Check sheet for the modelled part. Datum: model origin and axes. Units: mm. Face numbers are marked on the shaded views. A direction names the side the tool comes from. Coordinates: 2 decimals unless noted, no trailing zeros. Loops run counter-clockwise (first coordinate to the right, second up) from the corner with the lowest first, then second, coordinate; pieces in that order, holes last.
```python
from build123d import *

# Parameters (mm, degrees)
SKETCH1_W                = 72
SKETCH1_H                = 70
BOSS_EXTRUDE1_DEPTH      = 2
BOSS_EXTRUDE2_DEPTH      = 34
BOSS_EXTRUDE2_DEPTH_BACK = 34
CUT_EXTRUDE1_START       = -34
SKETCH3_W                = 39.5
SKETCH3_H                = 2
CUT_EXTRUDE1_DEPTH       = 68
BOSS_EXTRUDE3_DEPTH      = 2
FILLET2_R                = 1
FILLET2_OF_MIRROR1_R     = 1


with BuildPart() as part:
    # Sketch1 → Boss-Extrude1 (new body)
    with BuildSketch(Plane(origin=(0, 0, 0), x_dir=(1, 0, 0), z_dir=(0, 1, 0))):
        Rectangle(SKETCH1_W, SKETCH1_H)
    extrude(amount=BOSS_EXTRUDE1_DEPTH)

    # Sketch2 → Boss-Extrude2 (add, two sides: drawn at the far end of the back side and taken through both)
    with BuildSketch(Plane(origin=(0, 0, 0), x_dir=(0, 0, -1), z_dir=(1, 0, 0)).offset(-BOSS_EXTRUDE2_DEPTH_BACK)):
        with BuildLine():
            Line((-25.991933385, 2), (-19.75, 2))
            Line((-19.75, 2), (-19.75, 6.5))
            ThreePointArc((-19.75, 6.5), (-13.763212024, 15.155284356), (-3.552389776, 12.606816862))
            Line((-3.552389776, 12.606816862), (3.552389776, 12.606816862))
            ThreePointArc((3.552389776, 12.606816862), (13.763212024, 15.155284356), (19.75, 6.5))
            Line((19.75, 6.5), (19.75, 2))
            Line((19.75, 2), (25.991933385, 2))
            ThreePointArc((25.991933385, 2), (22.513891667, 3.407893959), (20.994535519, 6.838709677))
            ThreePointArc((20.994535519, 6.838709677), (15.537625909, 15.712617717), (5.12195122, 15.51812571))
            ThreePointArc((5.12195122, 15.51812571), (0, 14.106816862), (-5.12195122, 15.51812571))
            ThreePointArc((-5.12195122, 15.51812571), (-15.537625909, 15.712617717), (-20.994535519, 6.838709677))
            ThreePointArc((-20.994535519, 6.838709677), (-22.513891667, 3.407893959), (-25.991933385, 2))
        make_face()
    extrude(amount=BOSS_EXTRUDE2_DEPTH + BOSS_EXTRUDE2_DEPTH_BACK)

    # Sketch3 → Cut-Extrude1 (cut)
    with BuildSketch(Plane(origin=(0, 0, 0), x_dir=(0, 0, -1), z_dir=(1, 0, 0)).offset(CUT_EXTRUDE1_START)):
        with Locations((0, 1)):
            Rectangle(SKETCH3_W, SKETCH3_H)
    extrude(amount=CUT_EXTRUDE1_DEPTH, mode=Mode.SUBTRACT)

    # Sketch4 → Boss-Extrude3 (add)
    with BuildSketch(Plane(origin=(34, 0, 0), x_dir=(0, 0, -1), z_dir=(1, 0, 0))):
        with BuildLine():
            Line((-25.991933385, 2), (25.991933385, 2))
            ThreePointArc((25.991933385, 2), (22.513891667, 3.407893959), (20.994535519, 6.838709677))
            ThreePointArc((20.994535519, 6.838709677), (15.537625909, 15.712617717), (5.12195122, 15.51812571))
            ThreePointArc((5.12195122, 15.51812571), (0, 14.106816862), (-5.12195122, 15.51812571))
            ThreePointArc((-5.12195122, 15.51812571), (-15.537625909, 15.712617717), (-20.994535519, 6.838709677))
            ThreePointArc((-20.994535519, 6.838709677), (-22.513891667, 3.407893959), (-25.991933385, 2))
        make_face()
    boss_extrude3 = extrude(amount=BOSS_EXTRUDE3_DEPTH)

    # Fillet2
    fillet2_edges = [part.edges().sort_by_distance(p)[0] for p in [
        (36, 2, 30.495966692),
        (36, 2, -30.495966692),
        (36, 3.407893959, -22.513891667),
        (36, 15.712617717, -15.537625909),
        (36, 14.106816862, 0),
        (36, 15.712617717, 15.537625909),
        (36, 3.407893959, 22.513891667),
    ]]
    fillet(fillet2_edges, radius=FILLET2_R)

    # Mirror1: Boss-Extrude3 across plane
    add(boss_extrude3.mirror(Plane(origin=(0, 0, 0), x_dir=(0, 0, 1), z_dir=(1, 0, 0))))

    # Fillet2 of Mirror1
    fillet2_of_mirror1_edges = [part.edges().sort_by_distance(p)[0] for p in [
        (-36, 2, 30.495966692),
        (-36, 2, -30.495966692),
        (-36, 3.407893959, -22.513891667),
        (-36, 15.712617717, -15.537625909),
        (-36, 14.106816862, 0),
        (-36, 15.712617717, 15.537625909),
        (-36, 3.407893959, 22.513891667),
    ]]
    fillet(fillet2_of_mirror1_edges, radius=FILLET2_OF_MIRROR1_R)


solid = part.part
```
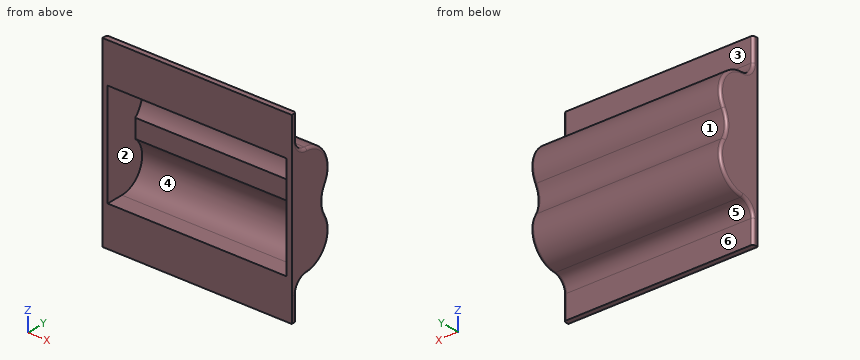
1) Depth check by flat-ended pin: pin 1 (5 mm diameter, centred on x = 20, y = 7, fed in from +Z); pin 2 (5 mm diameter, centred on x = -23.5, z = -26, fed in from +Y); pin 3 (2.5 mm diameter, centred on x = 0.5, z = 29.5, fed in from +Y). Enter the tip coordinate at first touch or a pass-through.
Answer sheet:
pin 1: stops at z = 21.66
pin 2: stops at y = 2.67
pin 3: stops at y = 2
2) Section check A-A on x = -1. Enter the section's corners in (y, z).
Answer sheet:
outline: (0, -35) - (2, -35) - (2, -25.99) arc R5 cw to (6.84, -20.99) arc R10.5 ccw to (15.52, -5.12) arc R10 cw to (15.52, 5.12) arc R10.5 ccw to (6.84, 20.99) arc R5 cw to (2, 25.99) - (2, 35) - (0, 35) - (0, 19.75) - (6.5, 19.75) arc R9.25 cw to (12.61, 3.55) - (12.61, -3.55) arc R9.25 cw to (6.5, -19.75) - (0, -19.75) - close
3) Scan lines: line 1 (X direction, y = 11.25, z = 14); line 2 (Z direction, x = 2.5, y = 1.25); line 3 (Z direction, x = 30, y = 12.75). Record each from-to range of solid material in increasing order.
Answer sheet:
line 1: x = -36 to -34, 34 to 36
line 2: z = -35 to -19.75, 19.75 to 35
line 3: z = -18.94 to -17.32, -3.68 to 3.68, 17.32 to 18.94
4) Set-up check for the marked faces 1, 2 and 3: record each of +Z, -Z, +X, -X, +Y, -Y from which the full face is reachable in a straight line by a thin tool's end or side.
Answer sheet:
face 1: +X, -X, +Y
face 2: -Y
face 3: +Z, +X, -X, +Y
5) Mould release check, pull along Z, two halves, no side actions. Record for the marked faces 4, 5 and 6: +Z half, -Z half, draft (parallel to the pull), parting line (faces both ways), or undercut.
Answer sheet:
face 4: undercut
face 5: -Z half
face 6: draft
6) Section check B-B on z = 29.5. Enter the section's corners in (x, y).
Answer sheet:
outline: (-36, 0) - (36, 0) - (36, 1) arc R1 ccw to (35, 2) - (-35, 2) arc R1 ccw to (-36, 1) - close
